from build123d import *

# Parameters (mm, degrees)
EXTRUDE_1_DEPTH          = 5
CUT_EXTRUDE_1_DEPTH      = 2
CUT_EXTRUDE_2_DEPTH      = 2
CUT_EXTRUDE_4_DEPTH      = 126.932521614
CUT_EXTRUDE_4_DEPTH_BACK = 126.932521614
SKETCH_6_R               = 1.5
SKETCH_7_R               = 1.5
CUT_EXTRUDE_5_DEPTH      = 126.932521614
CHAMFER_1_SIZE           = 0.5
CHAMFER_2_SIZE           = 0.5


with BuildPart() as part:
    # 草图1 → 凸台-拉伸1 (new body)
    with BuildSketch(Plane.XY):
        with BuildLine():
            Line((-110, 15), (110, 15))
            ThreePointArc((110, 15), (125, 0), (110, -15))
            Line((110, -15), (-110, -15))
            ThreePointArc((-110, -15), (-125, 0), (-110, 15))
        make_face()
    extrude(amount=EXTRUDE_1_DEPTH)

    # 草图2 → 切除-拉伸1 (cut)
    with BuildSketch(Plane.XY.offset(5)):
        with BuildLine():
            Line((114, 7), (114, -7))
            ThreePointArc((114, -7), (110, -11), (106, -7))
            Line((106, -7), (106, 7))
            ThreePointArc((106, 7), (110, 11), (114, 7))
        make_face()
        with BuildLine():
            Line((-106, 7), (-106, -7))
            ThreePointArc((-106, -7), (-110, -11), (-114, -7))
            Line((-114, -7), (-114, 7))
            ThreePointArc((-114, 7), (-110, 11), (-106, 7))
        make_face()
    extrude(amount=-CUT_EXTRUDE_1_DEPTH, mode=Mode.SUBTRACT)

    # 草图4 → 切除-拉伸2 (cut)
    with BuildSketch(Plane(origin=(0, 0, 0), x_dir=(-1, 0, 0), z_dir=(0, 0, -1))):
        with BuildLine():
            Line((-71.5, 7.5), (-71.5, -7.5))
            ThreePointArc((-71.5, -7.5), (-76.5, -12.5), (-81.5, -7.5))
            Line((-81.5, -7.5), (-81.5, 7.5))
            ThreePointArc((-81.5, 7.5), (-76.5, 12.5), (-71.5, 7.5))
        make_face()
        with BuildLine():
            Line((71.5, 7.5), (71.5, -7.5))
            ThreePointArc((71.5, -7.5), (76.5, -12.5), (81.5, -7.5))
            Line((81.5, -7.5), (81.5, 7.5))
            ThreePointArc((81.5, 7.5), (76.5, 12.5), (71.5, 7.5))
        make_face()
    extrude(amount=-CUT_EXTRUDE_2_DEPTH, mode=Mode.SUBTRACT)

    # 草图6 → 切除-拉伸4 (cut, two sides: drawn at the far end of the back side and taken through both)
    with BuildSketch(Plane(origin=(0, 0, 2), x_dir=(-1, 0, 0), z_dir=(0, 0, -1)).offset(-CUT_EXTRUDE_4_DEPTH_BACK)):
        with Locations((76.5, 7)):
            Circle(SKETCH_6_R)
        with Locations(Location((76.5, -7, 0), (0, 0, 180))):
            Circle(SKETCH_6_R)
        with Locations((-76.5, 7)):
            Circle(SKETCH_6_R)
        with Locations((-76.5, -7)):
            Circle(SKETCH_6_R)
    extrude(amount=CUT_EXTRUDE_4_DEPTH + CUT_EXTRUDE_4_DEPTH_BACK, mode=Mode.SUBTRACT)

    # 草图7 → 切除-拉伸5 (cut, through all)
    with BuildSketch(Plane.XY.offset(3)):
        with Locations((110, 7)):
            Circle(SKETCH_7_R)
        with Locations((110, -7)):
            Circle(SKETCH_7_R)
        with Locations((-110, 7)):
            Circle(SKETCH_7_R)
        with Locations((-110, -7)):
            Circle(SKETCH_7_R)
    extrude(amount=-CUT_EXTRUDE_5_DEPTH, mode=Mode.SUBTRACT)

    # 倒角1
    chamfer_1_edges = [part.edges().sort_by_distance(p)[0] for p in [
        (108.5, -7, 3),
        (-111.5, 7, 3),
        (-111.5, -7, 3),
        (108.5, 7, 3),
    ]]
    chamfer(chamfer_1_edges, length=CHAMFER_1_SIZE)

    # 倒角2
    chamfer_2_edges = [part.edges().sort_by_distance(p)[0] for p in [
        (-78, -7, 2),
        (78, 7, 2),
        (78, -7, 2),
        (-75, 7, 2),
    ]]
    chamfer(chamfer_2_edges, length=CHAMFER_2_SIZE)


solid = part.part
The model under review builds one solid part; all positions refer to its coordinate system, in mm. A direction names the side the tool comes from. Round coordinates to 2 decimals unless told otherwise and drop trailing zeros. Loops run counter-clockwise (first coordinate to the right, second up) from the corner with the lowest first, then second, coordinate; pieces in that order, holes last. Notation, with made-up numbers: M -33,-21 L -13,-21 A24 cw -13,12 Z; hole C 13,-31 d7. An arc over 180 degrees is marked long. Answer as a JSON object with one key per item and string values.
Item 1: Tool access review of faces 5 (the face through (110, -11, 4)), 6 (the face through (-76.6, 12.5, 1)), 7 (the face through (2, -15, 2)): name each direction out of +Z, -Z, +X, -X, +Y, -Y from which nothing blocks a thin tool from reaching the whole face with its end or side.
Check sheet entries:
{"face 5": "+Z", "face 6": "-Z", "face 7": "+Z, -Z, +X, -X, -Y"}
Item 2: The part is to be moulded in two halves that separate along Y. For faces 1 (the face through (-125, 0, 2)), 2 (the face through (76, 0, 2)), 3 (the face through (76.6, 12.5, 1)), 4 (the face through (-2, 15, 2)), say which applies: +Y half, -Y half, draft (parallel to the pull), parting line (faces both ways), or undercut.
Check sheet entries:
{"face 1": "parting line", "face 2": "undercut", "face 3": "undercut", "face 4": "+Y half"}
Item 3: We need section A-A, the plane y = 0. State the section outline as (x, z) points.
Check sheet entries:
{"outline": "M -125,0 L -81.5,0 L -81.5,2 L -71.5,2 L -71.5,0 L 71.5,0 L 71.5,2 L 81.5,2 L 81.5,0 L 125,0 L 125,5 L 114,5 L 114,3 L 106,3 L 106,5 L -106,5 L -106,3 L -114,3 L -114,5 L -125,5 Z"}
Item 4: Clearance check with flat-ended pins moving along their axes: P1, Ø5, axis at x = 76.5, y = 7, coming from the -Z side; P2, Ø3.5, axis at x = 76.5, y = -7, coming from the -Z side; P3, Ø1.6, axis at y = 3.5, z = 0.5, coming from the +X side (3 decimals); P4, Ø4, axis at x = -110, y = -7, coming from the -Z side. State where each tip first meets the part, or that it passes through.
Check sheet entries:
{"P1": "z = 2", "P2": "z = 2.25", "P3": "x = 124.755", "P4": "z = 0"}
Item 5: For line 1 along Y through (x, z) = (76.5, 3.25); line 2 along X through (y, z) = (6.5, 1.55); line 3 along X through (y, z) = (2, 4.25), list the stretches that pass through material, from the lowest coordinate up.
Check sheet entries:
{"line 1": "-15 to -8.5, -5.5 to 5.5, 8.5 to 15", "line 2": "-123.52 to -111.41, -108.59 to -81.5, -71.5 to 71.5, 81.5 to 108.59, 111.41 to 123.52", "line 3": "-124.87 to -114, -106 to 106, 114 to 124.87"}
